Autodesk Inventor part; units mm, degrees
ref_plane "YZ Plane" through (0, 0, 0) normal (1, 0, 0) x (0, 1, 0)
ref_plane "XZ Plane" through (0, 0, 0) normal (0, 1, 0) x (-1, 0, 0)
ref_plane "XY Plane" through (0, 0, 0) normal (0, 0, 1) x (1, 0, 0)
sketch "Sketch1" plane through (0, 0, 0) normal (0, 1, 0) x (-1, 0, 0)
  circle A0 centre (0, 0) radius 1.9812
  line L0 (6.35, 3.6662) -> (6.35, -3.6662)
  line L1 (6.35, -3.6662) -> (0, -7.3323)
  line L2 (0, -7.3323) -> (-6.35, -3.6662)
  line L3 (-6.35, -3.6662) -> (-6.35, 3.6662)
  line L4 (-6.35, 3.6662) -> (0, 7.3323)
  line L5 (0, 7.3323) -> (6.35, 3.6662)
  dimension "d0" = 3.9624
  dimension "d1" = 12.7
extrude "Extrusion1" add sketch "Sketch1" along normal blind 22.225
thread "Thread1"
properties part number "CLIM_007_HexHaft" material "Aluminum 6061"
Input: part model. Units: mm. Frame: model coordinates. Coordinates: 2 decimals unless noted, no trailing zeros. Write each loop counter-clockwise with the first axis right and the second up, starting at its lowest first coordinate (ties: lowest second). Pieces come first, ordered by that corner, then holes. Notation, with made-up numbers: M 60.25,68.5 L 117.25,68.5 A17 cw 117.25,90.5 Z; hole C 41,66.5 d5. An arc over 180 degrees is marked long. Answer as a JSON object with one key per item and string values. Group by question number.
(1) Contact query for flat-ended pins moving along their axis: P1, Ø4, axis at x = -2.5, y = 7.5, coming from the -Z side; P2, Ø5, axis at x = 5, y = 13.5, coming from the +Z side; P3, Ø3, axis at x = -2.5, y = 17, coming from the -Z side. Output: stop coordinate, or through.
(2) Section C-C on y = 6.5. Output: boundary loops of the cut face in (x, z), plus the area to 3 significant figures.
(3) Section B-B on x = 0.5. Output: boundary loops of the cut face in (y, z) (3 decimals).
(4) Section A-A on z = 0. Output: boundary loops of the cut face in (x, y) (3 decimals), plus the area to 3 significant figures.
(5) Ray query, line 1 along Z through (x, y) = (0.25, 8); line 2 along Z through (x, y) = (1.25, 18.75); line 3 along X through (y, z) = (18.25, 0.5). Return the intervals inside material, ascending. Write a range as [from, to].
(6) Mould query, pull axis X, two halves, no side actions, for faces 1 (the face through (0.258, 10.957, -1.964)), 2 (the face through (-3.131, 10.957, 5.525)), 3 (the face through (3.219, 10.957, 5.474)). Classes: pulls with the +X half, pulls with the -X half, needs draft (parallel to the pull), parting line crosses it, or undercut.
(7) Section D-D on z = 4. Output: boundary loops of the cut face in (x, y) (3 decimals), plus the area to 3 significant figures.
Result set:
{
 "1": {"P1": "stops at z = -7.04", "P2": "stops at z = 5.89", "P3": "stops at z = -6.75"},
 "2": {"outline": "M -6.35,-3.67 L 0,-7.33 L 6.35,-3.67 L 6.35,3.67 L 0,7.33 L -6.35,3.67 Z; hole C 0,0 d3.96", "area": "127 mm2"},
 "3": {"outline": "M 0,-7.044 L 22.225,-7.044 L 22.225,-1.917 L 0,-1.917 Z; M 0,1.917 L 22.225,1.917 L 22.225,7.044 L 0,7.044 Z"},
 "4": {"outline": "M -6.35,0 L -1.981,0 L -1.981,22.225 L -6.35,22.225 Z; M 1.981,0 L 6.35,0 L 6.35,22.225 L 1.981,22.225 Z", "area": "194 mm2"},
 "5": {"line 1": "z = [-7.19, -1.97], [1.97, 7.19]", "line 2": "z = [-6.61, -1.54], [1.54, 6.61]", "line 3": "x = [-6.35, -1.92], [1.92, 6.35]"},
 "6": {"face 1": "undercut", "face 2": "pulls with the -X half", "face 3": "pulls with the +X half"},
 "7": {"outline": "M -5.772,0 L 5.772,0 L 5.772,22.225 L -5.772,22.225 Z", "area": "257 mm2"}
}
